Autodesk Fusion 360 part; units mm, degrees
sketch "Walls" plane through (0, 0, 0) normal (0, 1, 0) x (1, 0, 0)
  line L0 (-80, 50) -> (80, 50)
  line L1 (90, 40) -> (90, -40)
  line L2 (80, -50) -> (-80, -50)
  line L3 (-90, -40) -> (-90, 40)
  line L4 (-90, 50) -> (90, -50) construction
  line L5 (90, 50) -> (-90, -50) construction
  arc A0 (-90, -40) -> (-80, -50) centre (-80, -40) ccw
  arc A1 (80, -50) -> (90, -40) centre (80, -40) ccw
  arc A2 (90, 40) -> (80, 50) centre (80, 40) ccw
  arc A3 (-80, 50) -> (-90, 40) centre (-80, 40) ccw
  arc A4 (87, 40) -> (80, 47) centre (80, 40) ccw
  line L6 (-80, 47) -> (80, 47)
  arc A5 (-80, 47) -> (-87, 40) centre (-80, 40) ccw
  line L7 (-87, -40) -> (-87, 40)
  arc A6 (-87, -40) -> (-80, -47) centre (-80, -40) ccw
  line L8 (80, -47) -> (-80, -47)
  arc A7 (80, -47) -> (87, -40) centre (80, -40) ccw
  line L9 (87, 40) -> (87, -40)
  dimension "d1" = 180
  dimension "d2" = 100
  dimension "d3" = 10
  dimension "d4" = 3
extrude "Floor Extrusion" add sketch "Walls" along normal blind 3 contours L0 L1 L2 L3 A0 A1 A2 A3 | A4 L6 A5 L7 A6 L8 A7 L9
extrude "Walls Extrusion" add sketch "Walls" along normal blind 15
sketch "Port" plane through (0, 0, -50) normal (0, 0, -1) x (-1, 0, 0)
  line L0 (-80, 0) -> (80, 0)
  line L1 (80, 0) -> (80, 15)
  line L2 (80, 15) -> (-80, 15)
  line L3 (-80, 15) -> (-80, 0)
  line L4 (4, 11.5) -> (-4, 11.5)
  arc A0 (-4, 11.5) -> (-4, 3.5) centre (-4, 7.5) ccw
  line L5 (-4, 3.5) -> (4, 3.5)
  arc A1 (4, 3.5) -> (4, 11.5) centre (4, 7.5) ccw
  line L6 (4, 7.5) -> (-4, 7.5) construction
  line L7 (80, 0) -> (-80, 0)
  dimension "d11" = 8
  dimension "d12" = 8
  dimension "d25" = 4
  dimension "d42" = 7.5
extrude "Port Extrusion" cut sketch "Port" against normal blind 3 contours L4 A0 L5 A1
sketch "Tab Holes" plane through (0, 0, 0) normal (1, 0, 0) x (0, 0, -1)
  circle A0 centre (0, 10) radius 1.25
  line L0 (-40, 15) -> (40, 15)
  dimension "d26" = 2.5
  dimension "d27" = 5
extrude "Tab Holes Extrusion" cut sketch "Tab Holes" along normal through all and the other way through all
sketch "Encoder Blocks" plane through (0, 3, 0) normal (0, 1, 0) x (-1, 0, 0)
  line L0 (87, -40) -> (87, 40)
  arc A0 (87, 40) -> (80, 47) centre (80, 40) ccw
  line L1 (80, 47) -> (-80, 47)
  arc A1 (-80, 47) -> (-87, 40) centre (-80, 40) ccw
  line L2 (-87, 40) -> (-87, -40)
  arc A2 (-87, -40) -> (-80, -47) centre (-80, -40) ccw
  line L3 (-80, -47) -> (80, -47)
  arc A3 (80, -47) -> (87, -40) centre (80, -40) ccw
  line L4 (73.8, -45) -> (56.8, -45)
  line L5 (56.8, -45) -> (56.8, -33)
  line L6 (56.8, -33) -> (73.8, -33)
  line L7 (73.8, -33) -> (73.8, -45)
  line L8 (73.8, -45) -> (56.8, -33) construction
  line L9 (56.8, -45) -> (73.8, -33) construction
  line L10 (80, -50) -> (-80, -50)
  line L11 (90, 40) -> (90, -40)
  line L12 (-56.8, -45) -> (-73.8, -33) construction
  line L13 (-56.8, -33) -> (-56.8, -45)
  line L14 (-56.8, -45) -> (-73.8, -45)
  line L15 (-73.8, -45) -> (-56.8, -33) construction
  line L16 (-73.8, -33) -> (-56.8, -33)
  line L17 (-73.8, -45) -> (-73.8, -33)
  line L18 (80, -47) -> (-80, -47)
  line L19 (-90, -40) -> (-90, 40)
  point P0 (65.3, -39)
  point P1 (-65.3, -39)
  dimension "d29" = 17
  dimension "d30" = 12
  dimension "d31" = 5
  dimension "d32" = 16.2
  dimension "d35" = 17
  dimension "d36" = 12
  dimension "d38" = 5
  dimension "d39" = 16.2
extrude "Left Encoder Block Extrusion" add sketch "Encoder Blocks" along normal blind 9 contours L4 L5 L6 L7
extrude "Right Encoder Block Extrusion" add sketch "Encoder Blocks" along normal blind 9 contours L13 L14 L16 L17
equation "d25 = ( 8 / 2 ) * 1 mm"
equation "d27 = ( 10 / 2 ) * 1 mm"
equation "d33 = 15 mm - 3 mm - 3 mm"
equation "d40 = 15 mm - 3 mm - 3 mm"
equation "d42 = ( 15 / 2 ) * 1 mm"
Source: CAD feature listing. Evaluate the final solid. Frame: model axes, mm. A direction names the side the tool comes from. Coordinates: 2 decimals unless noted, no trailing zeros. Order: outer loops, then holes, each group sorted by start corner. A loop starts at its lowest first (then second) coordinate and runs counter-clockwise, first axis right, second up. Notation, with made-up numbers: (-28.5, -34) - (-1.5, -34) arc R9 ccw to (-1.5, -21) - close; hole circle Ø4 at (-20, -17). An arc over 180 degrees is marked (long way). One line per item, written item: value.
1) Ray query, line 1 (Z direction, x = -77.5, y = 7.75); line 2 (X direction, y = 5.75, z = 12); line 3 (Z direction, x = -67.5, y = 9.5). Return the intervals inside material, ascending. Write a range as [from, to].
Computed values:
line 1: z = [-50, -47], [47, 50]
line 2: x = [-90, -87], [87, 90]
line 3: z = [-50, -47], [-45, -33], [47, 50]
2) Mould query, pull axis Z, two halves, no side actions, for faces 1 (the face through (86.99, 7.4, -47.15)), 2 (the face through (-1, 0, -1)), 3 (the face through (-65, 7, -45)). Classes: released by +Z, released by -Z, zero draft, split by the parting line, or undercut.
Computed values:
face 1: released by -Z
face 2: zero draft
face 3: undercut
3) Cut plane C-C on x = -30. Output: boundary loops of the cut face in (y, z).
Computed values:
outline: (0, -50) - (15, -50) - (15, -47) - (3, -47) - (3, 47) - (15, 47) - (15, 50) - (0, 50) - close
4) Contact query for flat-ended pins moving along their axis: pin 1 (3 mm diameter, centred on x = 30, z = -19.5, fed in from +Y); pin 2 (1.5 mm diameter, centred on y = 10, z = 0, fed in from +X); pin 3 (1 mm diameter, centred on x = -3.5, y = 10.5, fed in from -Z). Output: stop coordinate, or through.
Computed values:
pin 1: stops at y = 3
pin 2: passes through
pin 3: stops at z = 47
5) Cut plane B-B on z = 37.5. Output: boundary loops of the cut face in (x, y).
Computed values:
outline: (-90, 0) - (90, 0) - (90, 15) - (87, 15) - (87, 3) - (-87, 3) - (-87, 15) - (-90, 15) - close
6) Reachability of faces 4 (the face through (-86.99, 7.4, 47.15)), 5 (the face through (-8, 7.4, -48.5)), 6 (the face through (-84.9, 8.9, 45)) from +Z, -Z, +X, -X, +Y, -Y: full face, straight path, thin tool, end or side. Return the list, or none.
Computed values:
face 4: +Z, -X, +Y, -Y
face 5: -Z
face 6: +Y
7) Cut plane A-A on x = -65. Output: boundary loops of the cut face in (y, z), plus the area to 3 significant figures.
Computed values:
outline: (0, -50) - (15, -50) - (15, -47) - (3, -47) - (3, -45) - (12, -45) - (12, -33) - (3, -33) - (3, 47) - (15, 47) - (15, 50) - (0, 50) - close
area: 480 mm^2
